```python
from build123d import *

# Parameters (mm, degrees)
CROQUIS1_R                = 1.5875
SALIENTE_EXTRUIR1_DEPTH   = 6.5
SALIENTE_EXTRUIR1_2_DEPTH = 6.5
SALIENTE_EXTRUIR1_3_DEPTH = 6.5
SALIENTE_EXTRUIR1_4_DEPTH = 6.5
SALIENTE_EXTRUIR2_DEPTH   = 4.5
CROQUIS3_W                = 23
CROQUIS3_H                = 34
SALIENTE_EXTRUIR3_DEPTH   = 1


with BuildPart() as part:
    # Croquis1 → Saliente-Extruir1 (new body)
    with BuildSketch(Plane.XY):
        with Locations((14.790535489, 1.2625)):
            Circle(CROQUIS1_R)
    extrude(amount=SALIENTE_EXTRUIR1_DEPTH)



with BuildPart() as body_2:
    # Croquis1 → Saliente-Extruir1 2 (new body)
    with BuildSketch(Plane.XY):
        with Locations((14.790535489, -29.5625)):
            Circle(CROQUIS1_R)
    extrude(amount=SALIENTE_EXTRUIR1_2_DEPTH)


with BuildPart() as body_3:
    # Croquis1 → Saliente-Extruir1 3 (new body)
    with BuildSketch(Plane.XY):
        with Locations((-13.784464511, -29.5625)):
            Circle(CROQUIS1_R)
    extrude(amount=SALIENTE_EXTRUIR1_3_DEPTH)


with BuildPart() as body_4:
    # Croquis1 → Saliente-Extruir1 4 (new body)
    with BuildSketch(Plane.XY):
        with Locations((-13.784464511, 1.2625)):
            Circle(CROQUIS1_R)
    extrude(amount=SALIENTE_EXTRUIR1_4_DEPTH)


with BuildPart() as body_5:
    # Croquis2 → Saliente-Extruir2 (new body)
    with BuildSketch(Plane.XY.offset(2)):
        with BuildLine():
            ThreePointArc((-15.996964511, 5.35), (-17.411178073, 4.764213562), (-17.996964511, 3.35))
            Line((-17.996964511, 3.35), (-17.996964511, -31.65))
            ThreePointArc((-17.996964511, -31.65), (-17.411178073, -33.064213562), (-15.996964511, -33.65))
            Line((-15.996964511, -33.65), (17.003035489, -33.65))
            ThreePointArc((17.003035489, -33.65), (18.417249051, -33.064213562), (19.003035489, -31.65))
            Line((19.003035489, -31.65), (19.003035489, 3.35))
            ThreePointArc((19.003035489, 3.35), (18.417249051, 4.764213562), (17.003035489, 5.35))
            Line((17.003035489, 5.35), (-15.996964511, 5.35))
        make_face()
        with BuildLine():
            Line((-16.496964511, -8.883114021), (-16.496964511, 3.85))
            Line((-16.496964511, 3.85), (17.503035489, 3.85))
            Line((17.503035489, 3.85), (17.503035489, -32.15))
            Line((17.503035489, -32.15), (-16.496964511, -32.15))
            Line((-16.496964511, -32.15), (-16.496964511, -19.416885979))
            ThreePointArc((-16.496964511, -19.416885979), (-16.73791903, -18.965158785), (-16.821172495, -18.46))
            Line((-16.821172495, -18.46), (-16.821172495, -9.84))
            ThreePointArc((-16.821172495, -9.84), (-16.73791903, -9.334841215), (-16.496964511, -8.883114021))
        make_face(mode=Mode.SUBTRACT)
    extrude(amount=SALIENTE_EXTRUIR2_DEPTH)


with BuildPart() as part_1:
    add(part.part)

    add(body_2.part)  # Saliente-Extruir3 merges body 2

    add(body_3.part)  # Saliente-Extruir3 merges body 3

    add(body_4.part)  # Saliente-Extruir3 merges body 4

    add(body_5.part)  # Saliente-Extruir3 merges body 5
    # Croquis3 → Saliente-Extruir3 (add)
    with BuildSketch(Plane.XY.offset(6.5)):
        with BuildLine():
            ThreePointArc((19.003035489, 3.35), (18.417249051, 4.764213562), (17.003035489, 5.35))
            Line((17.003035489, 5.35), (-15.996964511, 5.35))
            ThreePointArc((-15.996964511, 5.35), (-17.411178073, 4.764213562), (-17.996964511, 3.35))
            Line((-17.996964511, 3.35), (-17.996964511, -31.65))
            ThreePointArc((-17.996964511, -31.65), (-17.411178073, -33.064213562), (-15.996964511, -33.65))
            Line((-15.996964511, -33.65), (17.003035489, -33.65))
            ThreePointArc((17.003035489, -33.65), (18.417249051, -33.064213562), (19.003035489, -31.65))
            Line((19.003035489, -31.65), (19.003035489, 3.35))
        make_face()
        with BuildLine():
            ThreePointArc((-16.821172495, -9.84), (-16.73791903, -9.334841215), (-16.496964511, -8.883114021))
            Line((-16.496964511, -8.883114021), (-16.496964511, 3.85))
            Line((-16.496964511, 3.85), (17.503035489, 3.85))
            Line((17.503035489, 3.85), (17.503035489, -32.15))
            Line((17.503035489, -32.15), (-16.496964511, -32.15))
            Line((-16.496964511, -32.15), (-16.496964511, -19.416885979))
            ThreePointArc((-16.496964511, -19.416885979), (-16.73791903, -18.965158785), (-16.821172495, -18.46))
            Line((-16.821172495, -18.46), (-16.821172495, -9.84))
        make_face(mode=Mode.SUBTRACT)
        with BuildLine():
            Line((-16.496964511, -8.883114021), (-16.496964511, 3.85))
            Line((-16.496964511, 3.85), (17.503035489, 3.85))
            Line((17.503035489, 3.85), (17.503035489, -32.15))
            Line((17.503035489, -32.15), (-16.496964511, -32.15))
            Line((-16.496964511, -32.15), (-16.496964511, -19.416885979))
            ThreePointArc((-16.496964511, -19.416885979), (-16.73791903, -18.965158785), (-16.821172495, -18.46))
            Line((-16.821172495, -18.46), (-16.821172495, -9.84))
            ThreePointArc((-16.821172495, -9.84), (-16.73791903, -9.334841215), (-16.496964511, -8.883114021))
        make_face()
        with Locations((0.803035489, -14.15)):
            Rectangle(CROQUIS3_W, CROQUIS3_H, mode=Mode.SUBTRACT)
    extrude(amount=SALIENTE_EXTRUIR3_DEPTH)


solid = part_1.part
```
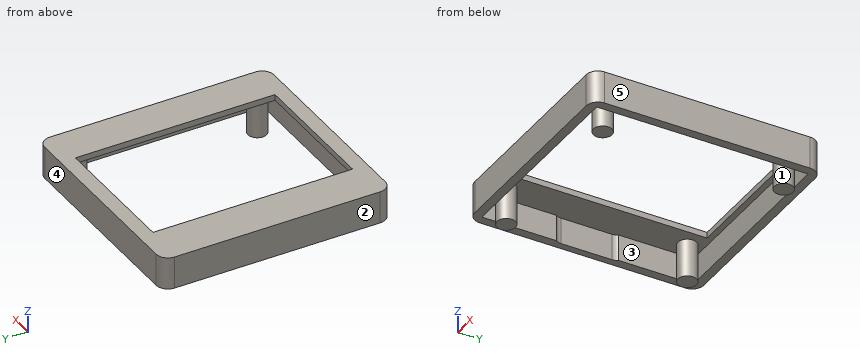
Source: CAD feature listing. Evaluate the final solid. Frame: model axes, mm. Face numbers are marked on the shaded views. A direction names the side the tool comes from. Coordinates: 2 decimals unless noted, no trailing zeros. Order: outer loops, then holes, each group sorted by start corner. A loop starts at its lowest first (then second) coordinate and runs counter-clockwise, first axis right, second up. Notation, with made-up numbers: M -24,32 L 32,32 A16 ccw 32,56 Z; hole C 0,-11 d11. An arc over 180 degrees is marked long. Write each question's results on one line, items separated by ' | '. Start each with the question number.
1) Section query B-B (z = 5.75). Give the number of separate pieces and of enclosed holes in the cut face, plus the area to 3 significant figures.
2) Section query A-A (y = -21). Return the cut outline in (x, z).
3) Access query for the marked faces 1 and 2. Directions: +Z, -Z, +X, -X, +Y, -Y. A direction counts if a zero-diameter tool reaches every point of the face in a straight line with its end or side. Return the directions, or none.
4) Section query D-D (y = -30.5). Return the cut outline in (x, z), plus the area to 3 significant figures.
5) Section query C-C (x = -4). Return the cut outline in (y, z).
6) Line query: line 1 (Y direction, x = -4, z = 4.5); line 2 (X direction, y = 2, z = 5.75); line 3 (X direction, y = -3, z = 7). Output: solid intervals per line, ascending. Write a range as from..to.
7) Contact query for flat-ended pins moving along their axis: pin 1 Ø18.5 at (x, y) = (-6, -11.5) entering from -Z; pin 2 Ø8 at (x, y) = (3.5, 1.5) entering from -Z. Output: stop coordinate, or through.
8) Draft query along X for the marked faces 3, 4 and 5. Return one class per face: released by +X, released by -X, zero draft, split by the parting line, or undercut.
Answers:
1) separate pieces: 5 | enclosed holes: 1 | area: 244 mm^2
2) outline: M -18,2 L -16.5,2 L -16.5,6.5 L -10.7,6.5 L -10.7,7.5 L -18,7.5 Z; M 12.3,6.5 L 17.5,6.5 L 17.5,2 L 19,2 L 19,7.5 L 12.3,7.5 Z
3) face 1: -Z | face 2: +Z, -Z, -X, +Y, -Y
4) outline: M -18,2 L -16.5,2 L -16.5,6.5 L -15.07,6.5 L -15.07,0 L -12.5,0 L -12.5,6.5 L -10.7,6.5 L -10.7,7.5 L -18,7.5 Z; M 12.3,6.5 L 13.51,6.5 L 13.51,0 L 16.07,0 L 16.07,6.5 L 17.5,6.5 L 17.5,2 L 19,2 L 19,7.5 L 12.3,7.5 Z | area: 60.8 mm^2
5) outline: M -33.65,2 L -32.15,2 L -32.15,6.5 L -31.15,6.5 L -31.15,7.5 L -33.65,7.5 Z; M 2.85,6.5 L 3.85,6.5 L 3.85,2 L 5.35,2 L 5.35,7.5 L 2.85,7.5 Z
6) line 1: y = -33.65..-32.15, 3.85..5.35 | line 2: x = -18..-16.5, -15.19..-12.38, 13.38..16.2, 17.5..19 | line 3: x = -18..-10.7, 12.3..19
7) pin 1: stops at z = 6.5 | pin 2: stops at z = 2
8) face 3: undercut | face 4: zero draft | face 5: released by +X
